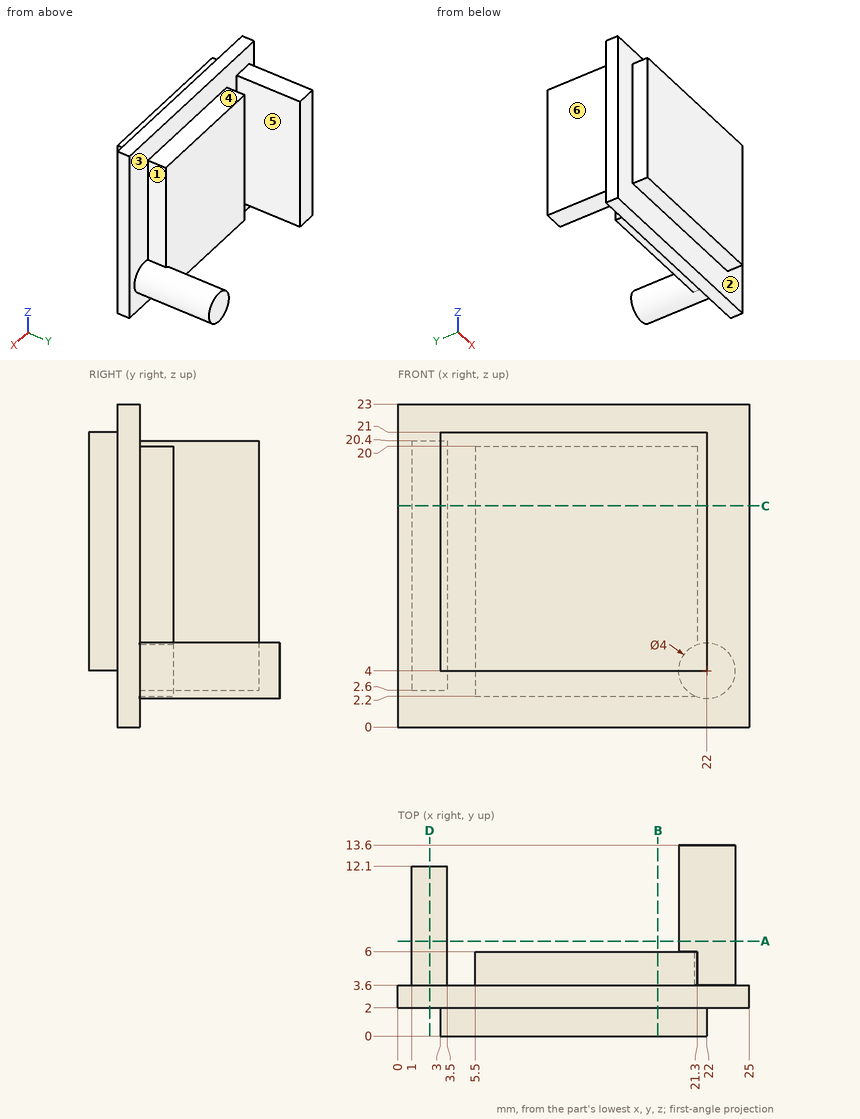
Source: three-view drawing plus pictorial views. Frame: mm from the lowest corner of the part. A direction names the side the tool comes from. Round coordinates to 2 decimals unless told otherwise and drop trailing zeros. Order: outer loops, then holes, each group sorted by start corner. A loop starts at its lowest first (then second) coordinate and runs counter-clockwise, first axis right, second up. Notation, with made-up numbers: (-39, -38.75) -> (-11, -38.75) arc R34 cw to (-11, -4.75) -> close; hole circle Ø11 at (-7.75, 26.25). An arc over 180 degrees is marked (long way). Use CSV: the item, a comma, the result in double quotes. Start each with the question number.
1) Section C-C (z = 15.75). Return the cut outline in (x, y), and give its area (3 significant figures).
2) First-contact query: pin 1 Ø6 at (x, z) = (6.5, 4.5) entering from -Y; pin 2 Ø1.2 at (x, z) = (2.5, 15.5) entering from +Y; pin 3 Ø3 at (x, y) = (7, 6.5) entering from +Z; pin 4 Ø10 at (x, z) = (16.5, 17) entering from +Y. Flat tips, straight axial feed; report the tip coordinate or a pass-through.
3) Section A-A (y = 6.75). Return the cut outline in (x, z), and give its area (3 significant figures).
4) Section D-D (x = 2.25). Return the cut outline in (y, z).
5) Draft query along X for the marked faces 1, 2 and 3. Return one class per face: +X half, -X half, draft (parallel to the pull), parting line (faces both ways), or undercut.
6) Section B-B (x = 18.5). Return the cut outline in (y, z).
7) Set-up query: the marked faces 4, 5 and 6. Return all of +Z, -Z, +X, -X, +Y, -Y with unobstructed straight access to the full face (end or side cutting, diameter ignored); none if empty.
8) Material intervals for line 1 along X through (y, z) = (5.75, 17.5); line 2 along Y through (x, z) = (20, 18.5); line 3 along Y through (x, z) = (12.75, 21.5), sorted ascending. Write a range as from..to.
Returned:
1,outline,"(0, 2) -> (3, 2) -> (3, 0) -> (22, 0) -> (22, 2) -> (25, 2) -> (25, 3.6) -> (21.3, 3.6) -> (21.3, 6) -> (5.5, 6) -> (5.5, 3.6) -> (3.5, 3.6) -> (3.5, 12.1) -> (1, 12.1) -> (1, 3.6) -> (0, 3.6) -> close"
1,area,"137 mm²"
2,pin 1,"stops at y = 0"
2,pin 2,"stops at y = 12.1"
2,pin 3,"stops at z = 20"
2,pin 4,"stops at y = 6"
3,outline,"(1, 2.6) -> (3.5, 2.6) -> (3.5, 20.4) -> (1, 20.4) -> close; circle Ø4 at (22, 4)"
3,area,"57.1 mm²"
4,outline,"(2, 0) -> (3.6, 0) -> (3.6, 2.6) -> (12.1, 2.6) -> (12.1, 20.4) -> (3.6, 20.4) -> (3.6, 23) -> (2, 23) -> close"
5,face 1,"+X half"
5,face 2,"draft"
5,face 3,"undercut"
6,outline,"(0, 4) -> (2, 4) -> (2, 0) -> (3.6, 0) -> (3.6, 2.2) -> (6, 2.2) -> (6, 20) -> (3.6, 20) -> (3.6, 23) -> (2, 23) -> (2, 21) -> (0, 21) -> close"
7,face 4,"+Z, +X, +Y"
7,face 5,"+Z, -Z, +Y"
7,face 6,"+Z, -Z, -X, +Y"
8,line 1,"x = 1..3.5, 5.5..21.3"
8,line 2,"y = 0..6"
8,line 3,"y = 2..3.6"
